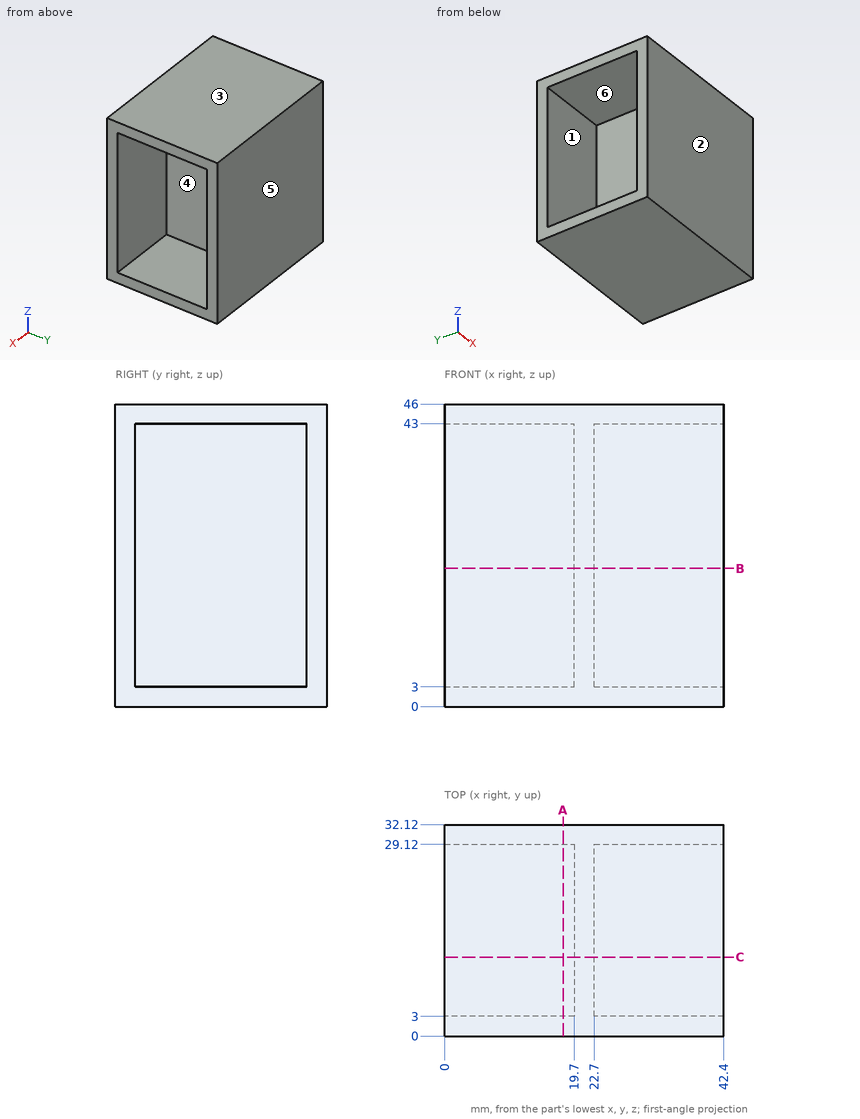
The figure shows three views and two pictorial views of one solid part (mm, origin at its lowest corner). Answer the questions. A direction names the side the tool comes from. Give positions to 0.01 mm unless a question says otherwise; leave off trailing zeros. Order: outer loops, then holes, each group sorted by start corner. A loop starts at its lowest first (then second) coordinate and runs counter-clockwise, first axis right, second up. Notation, with made-up numbers: (-39, 59.5) -> (-34, 59.5) arc R30 cw to (-34, 95.5) -> close; hole circle Ø10 at (65.5, -9.5). An arc over 180 degrees is marked (long way). Answer as CSV lines item,"result". Start each with the question number.
(1) This flat-tipped pin is pushed along its axis until it touches: pin 1 Ø3 at (y, z) = (18.5, 33.5) entering from +X. Where does it stop, or does it pass through?
(2) Section A-A, the plane x = 18 is taken. Write down the section's boundary in (y, z).
(3) For a pull along Y with two mould halves and no side action, classify the marked faces 1, 2 and 3 as released by +Y, released by -Y, zero draft, split by the parting line, or undercut.
(4) Section C-C, the plane y = 12 is taken. Write down the section's boundary in (x, z).
(5) Consider line 1 along Z through (x, y) = (11, 24); line 2 along Y through (x, z) = (12, 6.5); line 3 along X through (y, z) = (17.5, 27). Determine where each line is inside the solid, lowest interval first.
(6) Which of the six approach directions +Z, -Z, +X, -X, +Y, -Y give full straight-line access (tool end or side, diameter ignored) to the marked faces 4, 5 and 6?
(7) Section B-B, the plane z = 21 is taken. Write down the section's boundary in (x, y), plus the area to 3 significant figures.
Entries:
1,pin 1,"x = 22.7"
2,outline,"(0, 0) -> (32.12, 0) -> (32.12, 46) -> (0, 46) -> close; hole (3, 3) -> (29.12, 3) -> (29.12, 43) -> (3, 43) -> close"
3,face 1,"undercut"
3,face 2,"released by -Y"
3,face 3,"zero draft"
4,outline,"(0, 0) -> (42.4, 0) -> (42.4, 3) -> (22.7, 3) -> (22.7, 43) -> (42.4, 43) -> (42.4, 46) -> (0, 46) -> (0, 43) -> (19.7, 43) -> (19.7, 3) -> (0, 3) -> close"
5,line 1,"0 to 3, 43 to 46"
5,line 2,"0 to 3, 29.12 to 32.12"
5,line 3,"19.7 to 22.7"
6,face 4,"+X"
6,face 5,"+Z, -Z, +X, -X, +Y"
6,face 6,"-X"
7,outline,"(0, 0) -> (42.4, 0) -> (42.4, 3) -> (22.7, 3) -> (22.7, 29.12) -> (42.4, 29.12) -> (42.4, 32.12) -> (0, 32.12) -> (0, 29.12) -> (19.7, 29.12) -> (19.7, 3) -> (0, 3) -> close"
7,area,"333 mm²"
